Autodesk Inventor part; units mm, degrees
ref_plane "YZ Plane" through (0, 0, 0) normal (1, 0, 0) x (0, 1, 0)
ref_plane "XZ Plane" through (0, 0, 0) normal (0, 1, 0) x (-1, 0, 0)
ref_plane "XY Plane" through (0, 0, 0) normal (0, 0, 1) x (1, 0, 0)
sketch "Sketch1" plane through (0, 0, 0) normal (1, 0, 0) x (0, 1, 0)
  line L0 (6.1628, 9.8367) -> (-21.8372, 9.8367)
  line L1 (-21.8372, 9.8367) -> (-21.8372, -18.1633)
  line L2 (-21.8372, -18.1633) -> (6.1628, -18.1633)
  line L3 (6.1628, -18.1633) -> (6.1628, 9.8367)
  circle A0 centre (-7.8372, -4.1633) radius 6.55
  point P0 (0, 0)
  point P1 (2.1628, 5.8367)
  point P2 (-17.8372, 5.8367)
  point P3 (-17.8372, -14.1633)
  point P4 (2.1628, -14.1633)
  dimension "d0" = 28
  dimension "d1" = 28
  dimension "d2" = 20
  dimension "d3" = 20
  dimension "d4" = 4
  dimension "d5" = 4
  dimension "d6" = 14
  dimension "d7" = 14
  dimension "d8" = 13.1
extrude "Extrusion1" add sketch "Sketch1" along normal blind 9
hole "Hole1" at (0, 2.1628, 5.8367) at (0, -17.8372, 5.8367) at (0, -17.8372, -14.1633) at (0, 2.1628, -14.1633) direction (1, 0, 0) diameter 2.5 end through all
sketch "Sketch2" plane through (0, 0, 0) normal (-1, 0, 0) x (0, 0, 1)
  circle A0 centre (-14.1633, -17.8372) radius 1.25
  circle A1 centre (5.8367, 2.1628) radius 1.25
  circle A2 centre (5.8367, -17.8372) radius 1.25
  circle A3 centre (-14.1633, 2.1628) radius 1.25
  circle A4 centre (-4.1633, -7.8372) radius 6.55
  line L0 (9.8367, 6.1628) -> (9.8367, -21.8372)
  line L1 (-18.1633, 6.1628) -> (9.8367, 6.1628)
  line L2 (-18.1633, -21.8372) -> (-18.1633, 6.1628)
  line L3 (9.8367, -21.8372) -> (-18.1633, -21.8372)
  circle A5 centre (-4.1633, -7.8372) radius 5.55
  point P0 (0, 0)
  dimension "d18" = 1
extrude "Extrusion2" add sketch "Sketch2" against normal blind 1 contours A4
fillet "Fillet1" radius 2 4 edges at (4.5, -21.8372, 9.8367) (4.5, 6.1628, 9.8367) (4.5, -21.8372, -18.1633) (4.5, 6.1628, -18.1633)
chamfer "Chamfer1" distance 0.5 angle 45 1 edges at (9, -14.3872, -4.1633)
properties part number "3DP_PLA_X_axis_idler_bearing_block" material "ABS Plastic"
Build history of the part. All positions in model axes, mm. A direction names the side the tool comes from. Round coordinates to 2 decimals unless told otherwise and drop trailing zeros. Write each loop counter-clockwise with the first axis right and the second up, starting at its lowest first coordinate (ties: lowest second). Pieces come first, ordered by that corner, then holes. Notation, with made-up numbers: (-24, -37.75) -> (6, -37.75) arc R14 cw to (6, -31.75) -> close; hole circle Ø9 at (64, 81.5). An arc over 180 degrees is marked (long way). Put each result on its own line as item: value.
Item 1: Slice it at A-A, the plane z = -14. Give the cut face in (x, y).
Here are the results:
outline: (0, -21.84) -> (9, -21.84) -> (9, -19.08) -> (0, -19.08) -> close; (0, -16.6) -> (9, -16.6) -> (9, 0.92) -> (0, 0.92) -> close; (0, 3.4) -> (9, 3.4) -> (9, 6.16) -> (0, 6.16) -> close
Item 2: Tool access for faces 1 (the face through (4.563, -16.617, 5.566)), 2 (the face through (1, -6, -10)): list every direction of +Z, -Z, +X, -X, +Y, -Y with a clear straight run to the whole face (end or side of a thin tool).
Here are the results:
face 1: +X, -X
face 2: +X
Item 3: Wall check: probe 1 along Y at (x, z) = (4, -15.25); probe 2 along Z at (x, y) = (6.5, 3.25); probe 3 along Z at (x, y) = (4.75, 2.5). Give the ranges that are in metal, low to high. Write a range as from..to.
Here are the results:
probe 1: y = -21.84..-18.45, -17.22..1.55, 2.78..6.16
probe 2: z = -18.16..-14.78, -13.55..5.22, 6.45..9.84
probe 3: z = -18.16..-15.37, -12.96..4.63, 7.04..9.84
Item 4: Flat gauge pins, fed straight in: P1, Ø2, axis at y = -17.84, z = 5.84, coming from the +X side; P2, Ø3, axis at y = -17.84, z = -14.16, coming from the +X side. Where does each tip first touch, or does it go through?
Here are the results:
P1: passes through
P2: stops at x = 9
Item 5: Slice it at B-B, the plane x = 7.25. Give the cut face in (y, z).
Here are the results:
outline: (-21.84, -16.16) arc R2 ccw to (-19.84, -18.16) -> (4.16, -18.16) arc R2 ccw to (6.16, -16.16) -> (6.16, 7.84) arc R2 ccw to (4.16, 9.84) -> (-19.84, 9.84) arc R2 ccw to (-21.84, 7.84) -> close; hole circle Ø2.5 at (-17.84, -14.16); hole circle Ø2.5 at (-17.84, 5.84); hole circle Ø13.1 at (-7.84, -4.16); hole circle Ø2.5 at (2.16, -14.16); hole circle Ø2.5 at (2.16, 5.84)
Item 6: Two-plate mould, pull along Y, no slides. Class faces 3 (the face through (4.7, -14.38, -4.45)), 4 (the face through (4.56, -21.27, -17.56)), 5 (the face through (4.563, 5.561, -17.593)): pulls with the +Y half, pulls with the -Y half, needs draft (parallel to the pull), parting line crosses it, or undercut.
Here are the results:
face 3: undercut
face 4: pulls with the -Y half
face 5: pulls with the +Y half
